The listing builds one solid part. Answer for the finished solid, in the listing's coordinates (mm). A direction names the side the tool comes from. Coordinates: 2 decimals unless noted, no trailing zeros. Loops run counter-clockwise (first coordinate to the right, second up) from the corner with the lowest first, then second, coordinate; pieces in that order, holes last. Notation, with made-up numbers: (3, 27) - (56, 27) arc R10 ccw to (56, 44) - close; hole circle Ø5 at (27.5, 84.5). An arc over 180 degrees is marked (long way). Return JSON: item names as keys, results as strings. Group by question number.
1. Which of the six approach directions +Z, -Z, +X, -X, +Y, -Y give full straight-line access (tool end or side, diameter ignored) to faces 1 (the face through (-1, -4.3, -61)), 2 (the face through (-80, -2, -60))?
2. Section A-A (z = -8) is taken. Write down the section's boundary in (x, y).
3. Section D-D (x = 77.5) is taken. Write down the section's boundary in (y, z), and give its area (3 significant figures).
4. Find the intervals of material crossed by line 1 along X through (y, z) = (-2, 60.5); line 2 along X through (y, z) = (-0.9, 11.5); line 3 along Z through (x, y) = (-60.5, -3.55), in increasing order.
5. The mould has two halves that part along Z. Classify faces 3 (the face through (-100, -2, 1)), 4 (the face through (-97.15, -2.12, -66.99)), 5 (the face through (75, -2, -60)): pulls with the +Z half, pulls with the -Z half, needs draft (parallel to the pull), parting line crosses it, or undercut.
6. Section B-B (x = -8) is taken. Write down the section's boundary in (y, z), and give its area (3 significant figures).
7. Section C-C (y = -2.3) is taken. State how many separate pieces and enclosed holes the cut face has, and give its area (3 significant figures).
```python
from build123d import *

# Parameters (mm, degrees)
F0_W     = 5
F0_H     = 10
F1_DEPTH = 4.3


with BuildPart() as f1:
    # F0 (on Front) → F1 (new body)
    with BuildSketch(Plane.XZ):
        with BuildLine():
            Line((90, 70), (-90, 70))
            ThreePointArc((-90, 70), (-97.071068, 67.071068), (-100, 60))
            Line((-100, 60), (-100, -60))
            ThreePointArc((-100, -60), (-97.071068, -67.071068), (-90, -70))
            Line((-90, -70), (90, -70))
            ThreePointArc((90, -70), (97.071068, -67.071068), (100, -60))
            Line((100, -60), (100, 60))
            ThreePointArc((100, 60), (97.071068, 67.071068), (90, 70))
        make_face()
        with Locations((-77.5, -60)):
            Rectangle(F0_W, F0_H, mode=Mode.SUBTRACT)
        with Locations((77.5, -60)):
            Rectangle(F0_W, F0_H, mode=Mode.SUBTRACT)
        with Locations((-77.5, 60)):
            Rectangle(F0_W, F0_H, mode=Mode.SUBTRACT)
        with BuildLine():
            ThreePointArc((-80, 45), (-78.535534, 48.535534), (-75, 50))
            Line((-75, 50), (75, 50))
            ThreePointArc((75, 50), (78.535534, 48.535534), (80, 45))
            Line((80, 45), (80, -45))
            ThreePointArc((80, -45), (78.535534, -48.535534), (75, -50))
            Line((75, -50), (-75, -50))
            ThreePointArc((-75, -50), (-78.535534, -48.535534), (-80, -45))
            Line((-80, -45), (-80, 45))
        make_face(mode=Mode.SUBTRACT)
        with Locations((77.5, 60)):
            Rectangle(F0_W, F0_H, mode=Mode.SUBTRACT)
    extrude(amount=F1_DEPTH)


solid = f1.part
```
The answers:
{
 "1": {"face 1": "+Z, -Z, +X, -X, -Y", "face 2": "+Y, -Y"},
 "2": {"outline": "(-100, -4.3) - (-80, -4.3) - (-80, 0) - (-100, 0) - close; (80, -4.3) - (100, -4.3) - (100, 0) - (80, 0) - close"},
 "3": {"outline": "(-4.3, -70) - (0, -70) - (0, -65) - (-4.3, -65) - close; (-4.3, -55) - (0, -55) - (0, -49.33) - (-4.3, -49.33) - close; (-4.3, 49.33) - (0, 49.33) - (0, 55) - (-4.3, 55) - close; (-4.3, 65) - (0, 65) - (0, 70) - (-4.3, 70) - close", "area": "91.8 mm2"},
 "4": {"line 1": "x = -99.99 to -80, -75 to 75, 80 to 99.99", "line 2": "x = -100 to -80, 80 to 100", "line 3": "z = -70 to -50, 50 to 70"},
 "5": {"face 3": "needs draft", "face 4": "pulls with the -Z half", "face 5": "undercut"},
 "6": {"outline": "(-4.3, -70) - (0, -70) - (0, -50) - (-4.3, -50) - close; (-4.3, 50) - (0, 50) - (0, 70) - (-4.3, 70) - close", "area": "172 mm2"},
 "7": {"separate pieces": "1", "enclosed holes": "5", "area": "11,700 mm2"}
}
